The listing builds one solid part. Answer for the finished solid, in the listing's coordinates (mm). Face numbers are marked on the shaded views. A direction names the side the tool comes from. Coordinates: 2 decimals unless noted, no trailing zeros. Write each loop counter-clockwise with the first axis right and the second up, starting at its lowest first coordinate (ties: lowest second). Pieces come first, ordered by that corner, then holes. Notation, with made-up numbers: M 50,56 L 59,56 A29 ccw 59,76 Z; hole C 73,46 d4. An arc over 180 degrees is marked long. Answer as a JSON object with one key per item and string values. Group by question number.
from build123d import *

# Parameters (mm, degrees)
F1_DEPTH  = 2
F2_DEPTH  = 45.5
F4_DEPTH  = 5
F5_R      = 2
F6_R      = 5
F8_DEPTH  = 42.5
F9_R      = 3
F10_DEPTH = 47.501


with BuildPart() as f1:
    # F0 (on Top) → F1 (new body)
    with BuildSketch(Plane.XY):
        with BuildLine():
            ThreePointArc((4.2311346427, 10), (0, 13.850000456), (-4.2311346427, 10))
            Line((-4.2311346427, 10), (-3.2252907411, 10))
            ThreePointArc((-3.2252907411, 10), (0, 12.850000456), (3.2252907411, 10))
            Line((3.2252907411, 10), (4.2311346427, 10))
        make_face()
        with BuildLine():
            Line((3.2252907411, 10), (-3.2252907411, 10))
            ThreePointArc((-3.2252907411, 10), (-0.2003810013, 6.3561836525), (3.25, 9.600000456))
            ThreePointArc((3.25, 9.600000456), (3.2438168034, 9.8003814573), (3.2252907411, 10))
        make_face()
        with BuildLine():
            ThreePointArc((3.2252907411, 10), (0, 12.850000456), (-3.2252907411, 10))
            Line((-3.2252907411, 10), (3.2252907411, 10))
        make_face()
        with BuildLine():
            ThreePointArc((-2.9352384841, 6), (-0.7731344117, 3.3397464334), (0, 0))
            ThreePointArc((0, 0), (0.7731344117, 3.3397464334), (2.9352384841, 6))
            Line((2.9352384841, 6), (2.2588706729, 6))
            ThreePointArc((2.2588706729, 6), (0, 5.350000456), (-2.2588706729, 6))
            Line((-2.2588706729, 6), (-2.9352384841, 6))
        make_face()
        with BuildLine():
            ThreePointArc((2.9352384841, -6), (0.7731344117, -3.3397464334), (0, 0))
            ThreePointArc((0, 0), (-0.7731344117, -3.3397464334), (-2.9352384841, -6))
            Line((-2.9352384841, -6), (2.9352384841, -6))
        make_face()
        with BuildLine():
            ThreePointArc((-4.2311346427, 10), (-3.8118292524, 7.7205170826), (-2.2588706729, 6))
            Line((-2.2588706729, 6), (2.2588706729, 6))
            ThreePointArc((2.2588706729, 6), (3.7190523228, 7.543024564), (4.25, 9.600000456))
            ThreePointArc((4.25, 9.600000456), (4.2452810408, 9.8002225432), (4.2311346427, 10))
            Line((4.2311346427, 10), (3.2252907411, 10))
            ThreePointArc((3.2252907411, 10), (3.2438168034, 9.8003814573), (3.25, 9.600000456))
            ThreePointArc((3.25, 9.600000456), (-0.2003810013, 6.3561836525), (-3.2252907411, 10))
            Line((-3.2252907411, 10), (-4.2311346427, 10))
        make_face()
        with BuildLine():
            ThreePointArc((-2.9352384841, -6), (-0.7731344117, -3.3397464334), (0, 0))
            ThreePointArc((0, 0), (-0.7731344117, 3.3397464334), (-2.9352384841, 6))
            ThreePointArc((-2.9352384841, 6), (-14.6584577236, 2.8174766307), (-8.3490864524, -7.5629934211))
            ThreePointArc((-8.3490864524, -7.5629934211), (-7.6, -6.85), (-6.8509135476, -7.5629934211))
            ThreePointArc((-6.8509135476, -7.5629934211), (-4.7825233693, -7.0584577236), (-2.9352384841, -6))
        make_face()
        with BuildLine():
            ThreePointArc((2.9352384841, 6), (0.7731344117, 3.3397464334), (0, 0))
            ThreePointArc((0, 0), (0.7731344117, -3.3397464334), (2.9352384841, -6))
            ThreePointArc((2.9352384841, -6), (4.7825233693, -7.0584577236), (6.8509135476, -7.5629934211))
            ThreePointArc((6.8509135476, -7.5629934211), (7.6, -6.85), (8.3490864524, -7.5629934211))
            ThreePointArc((8.3490864524, -7.5629934211), (13.2326306926, -5.1023006067), (15.2, 0))
            ThreePointArc((15.2, 0), (10.9397464334, 6.8268655883), (2.9352384841, 6))
        make_face()
        with BuildLine():
            ThreePointArc((-8.3490864524, -7.5629934211), (-14.6584577236, 2.8174766307), (-2.9352384841, 6))
            Line((-2.9352384841, 6), (-2.2588706729, 6))
            ThreePointArc((-2.2588706729, 6), (-3.8118292524, 7.7205170826), (-4.2311346427, 10))
            Line((-4.2311346427, 10), (-17.5, 10))
            Line((-17.5, 10), (-17.5, -10))
            Line((-17.5, -10), (17.5, -10))
            Line((17.5, -10), (17.5, 10))
            Line((17.5, 10), (4.2311346427, 10))
            ThreePointArc((4.2311346427, 10), (4.2452810408, 9.8002225432), (4.25, 9.600000456))
            ThreePointArc((4.25, 9.600000456), (3.7190523228, 7.543024564), (2.2588706729, 6))
            Line((2.2588706729, 6), (2.9352384841, 6))
            ThreePointArc((2.9352384841, 6), (10.9397464334, 6.8268655883), (15.2, 0))
            ThreePointArc((15.2, 0), (13.2326306926, -5.1023006067), (8.3490864524, -7.5629934211))
            ThreePointArc((8.3490864524, -7.5629934211), (8.3497715783, -7.5814910734), (8.35, -7.6))
            ThreePointArc((8.35, -7.6), (7.5814910734, -8.3497715783), (6.8509135476, -7.5629934211))
            ThreePointArc((6.8509135476, -7.5629934211), (4.7825233693, -7.0584577236), (2.9352384841, -6))
            Line((2.9352384841, -6), (-2.9352384841, -6))
            ThreePointArc((-2.9352384841, -6), (-4.7825233693, -7.0584577236), (-6.8509135476, -7.5629934211))
            ThreePointArc((-6.8509135476, -7.5629934211), (-6.8502284217, -7.5814910734), (-6.85, -7.6))
            ThreePointArc((-6.85, -7.6), (-7.6185089266, -8.3497715783), (-8.3490864524, -7.5629934211))
        make_face()
        with BuildLine():
            ThreePointArc((-6.8509135476, -7.5629934211), (-7.6, -6.85), (-8.3490864524, -7.5629934211))
            ThreePointArc((-8.3490864524, -7.5629934211), (-7.6, -7.6), (-6.8509135476, -7.5629934211))
        make_face()
        with BuildLine():
            ThreePointArc((-6.8509135476, -7.5629934211), (-7.6, -7.6), (-8.3490864524, -7.5629934211))
            ThreePointArc((-8.3490864524, -7.5629934211), (-7.6185089266, -8.3497715783), (-6.85, -7.6))
            ThreePointArc((-6.85, -7.6), (-6.8502284217, -7.5814910734), (-6.8509135476, -7.5629934211))
        make_face()
        with BuildLine():
            ThreePointArc((8.3490864524, -7.5629934211), (7.6, -6.85), (6.8509135476, -7.5629934211))
            ThreePointArc((6.8509135476, -7.5629934211), (7.6, -7.6), (8.3490864524, -7.5629934211))
        make_face()
        with BuildLine():
            ThreePointArc((8.3490864524, -7.5629934211), (7.6, -7.6), (6.8509135476, -7.5629934211))
            ThreePointArc((6.8509135476, -7.5629934211), (7.5814910734, -8.3497715783), (8.35, -7.6))
            ThreePointArc((8.35, -7.6), (8.3497715783, -7.5814910734), (8.3490864524, -7.5629934211))
        make_face()
        with BuildLine():
            Line((2.2588706729, 6), (-2.2588706729, 6))
            ThreePointArc((-2.2588706729, 6), (0, 5.350000456), (2.2588706729, 6))
        make_face()
    extrude(amount=-F1_DEPTH)

    # F0 (on Top) → F2 (join)
    with BuildSketch(Plane.XY):
        with BuildLine():
            ThreePointArc((-8.3490864524, -7.5629934211), (-14.6584577236, 2.8174766307), (-2.9352384841, 6))
            Line((-2.9352384841, 6), (-2.2588706729, 6))
            ThreePointArc((-2.2588706729, 6), (-3.8118292524, 7.7205170826), (-4.2311346427, 10))
            Line((-4.2311346427, 10), (-17.5, 10))
            Line((-17.5, 10), (-17.5, -10))
            Line((-17.5, -10), (17.5, -10))
            Line((17.5, -10), (17.5, 10))
            Line((17.5, 10), (4.2311346427, 10))
            ThreePointArc((4.2311346427, 10), (4.2452810408, 9.8002225432), (4.25, 9.600000456))
            ThreePointArc((4.25, 9.600000456), (3.7190523228, 7.543024564), (2.2588706729, 6))
            Line((2.2588706729, 6), (2.9352384841, 6))
            ThreePointArc((2.9352384841, 6), (10.9397464334, 6.8268655883), (15.2, 0))
            ThreePointArc((15.2, 0), (13.2326306926, -5.1023006067), (8.3490864524, -7.5629934211))
            ThreePointArc((8.3490864524, -7.5629934211), (8.3497715783, -7.5814910734), (8.35, -7.6))
            ThreePointArc((8.35, -7.6), (7.5814910734, -8.3497715783), (6.8509135476, -7.5629934211))
            ThreePointArc((6.8509135476, -7.5629934211), (4.7825233693, -7.0584577236), (2.9352384841, -6))
            Line((2.9352384841, -6), (-2.9352384841, -6))
            ThreePointArc((-2.9352384841, -6), (-4.7825233693, -7.0584577236), (-6.8509135476, -7.5629934211))
            ThreePointArc((-6.8509135476, -7.5629934211), (-6.8502284217, -7.5814910734), (-6.85, -7.6))
            ThreePointArc((-6.85, -7.6), (-7.6185089266, -8.3497715783), (-8.3490864524, -7.5629934211))
        make_face()
        with BuildLine():
            ThreePointArc((4.2311346427, 10), (0, 13.850000456), (-4.2311346427, 10))
            Line((-4.2311346427, 10), (-3.2252907411, 10))
            ThreePointArc((-3.2252907411, 10), (0, 12.850000456), (3.2252907411, 10))
            Line((3.2252907411, 10), (4.2311346427, 10))
        make_face()
        with BuildLine():
            ThreePointArc((-4.2311346427, 10), (-3.8118292524, 7.7205170826), (-2.2588706729, 6))
            Line((-2.2588706729, 6), (2.2588706729, 6))
            ThreePointArc((2.2588706729, 6), (3.7190523228, 7.543024564), (4.25, 9.600000456))
            ThreePointArc((4.25, 9.600000456), (4.2452810408, 9.8002225432), (4.2311346427, 10))
            Line((4.2311346427, 10), (3.2252907411, 10))
            ThreePointArc((3.2252907411, 10), (3.2438168034, 9.8003814573), (3.25, 9.600000456))
            ThreePointArc((3.25, 9.600000456), (-0.2003810013, 6.3561836525), (-3.2252907411, 10))
            Line((-3.2252907411, 10), (-4.2311346427, 10))
        make_face()
    extrude(amount=F2_DEPTH)

    # F3 (on face) → F4 (cut)
    with BuildSketch(Plane.XY.offset(45.5)):
        with BuildLine():
            ThreePointArc((4.2311346427, 10), (0, 13.850000456), (-4.2311346427, 10))
            Line((-4.2311346427, 10), (-17.5, 10))
            Line((-17.5, 10), (-17.5, -10))
            Line((-17.5, -10), (17.5, -10))
            Line((17.5, -10), (17.5, 10))
            Line((17.5, 10), (4.2311346427, 10))
        make_face()
        with BuildLine():
            Line((3.6523963674, 8.75), (16.25, 8.75))
            Line((16.25, 8.75), (16.25, -8.75))
            Line((16.25, -8.75), (-16.25, -8.75))
            Line((-16.25, -8.75), (-16.25, 8.75))
            Line((-16.25, 8.75), (-3.6523963674, 8.75))
            ThreePointArc((-3.6523963674, 8.75), (-0.4277929535, 13.3255196398), (3.75, 9.600000456))
            ThreePointArc((3.75, 9.600000456), (3.7255191838, 9.1722075025), (3.6523963674, 8.75))
        make_face(mode=Mode.SUBTRACT)
    extrude(amount=-F4_DEPTH, mode=Mode.SUBTRACT)

    # F5
    f5_edges = [f1.edges().sort_by_distance(p)[0] for p in [
        (17.5, -10, 19.25),
        (17.5, 10, 19.25),
        (-17.5, 10, 19.25),
        (-17.5, -10, 19.25),
    ]]
    fillet(f5_edges, radius=F5_R)

    # F6
    f6_edges = [f1.edges().sort_by_distance(p)[0] for p in [
        (16.25, -8.75, 43),
        (16.25, 8.75, 43),
        (-16.25, 8.75, 43),
        (-16.25, -8.75, 43),
    ]]
    fillet(f6_edges, radius=F6_R)

    # F7 (on face) → F8 (join)
    with BuildSketch(Plane(origin=(0, 0, -2), x_dir=(1, 0, 0), z_dir=(0, 0, -1))):
        with BuildLine():
            ThreePointArc((17.5, 0), (21.5, 4), (25.5, 0))
            ThreePointArc((25.5, 0), (25.0480433512, -1.8469944174), (23.794305811, -3.2766081312))
            ThreePointArc((23.794305811, -3.2766081312), (25.0884620929, -3.1917847095), (25.7612762908, -4.3005482325))
            ThreePointArc((25.7612762908, -4.3005482325), (25.6200398184, -4.8777340259), (25.2282467868, -5.3244883225))
            ThreePointArc((25.2282467868, -5.3244883225), (27.2655704017, -3.0013660128), (28, 0))
            ThreePointArc((28, 0), (24.3504385627, 5.8416607228), (17.5, 5.123475383))
            Line((17.5, 5.123475383), (17.5, 0))
        make_face()
        with BuildLine():
            ThreePointArc((25.7612762908, -4.3005482325), (25.0884620929, -3.1917847095), (23.794305811, -3.2766081312))
            ThreePointArc((23.794305811, -3.2766081312), (23.4873361952, -5.0175187204), (25.2282467868, -5.3244883225))
            ThreePointArc((25.2282467868, -5.3244883225), (25.6200398184, -4.8777340259), (25.7612762908, -4.3005482325))
        make_face()
    extrude(amount=-F8_DEPTH)

    # F9 (on face) → F10 (cut, through all)
    with BuildSketch(Plane(origin=(0, 0, -2), x_dir=(1, 0, 0), z_dir=(0, 0, -1))):
        with Locations((0, -9.600000456)):
            Circle(F9_R)
    extrude(amount=-F10_DEPTH, mode=Mode.SUBTRACT)


solid = f1.part
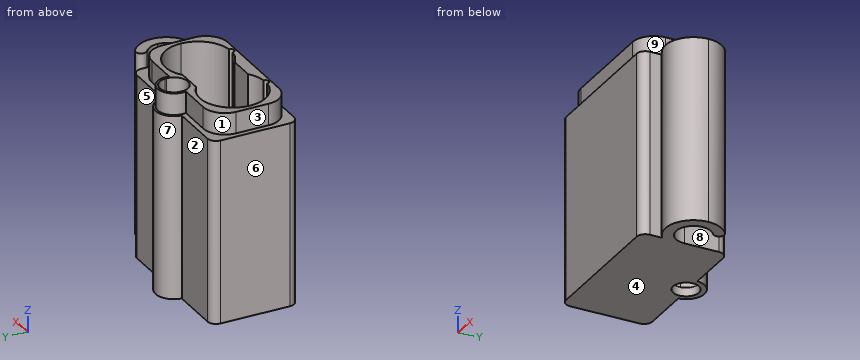
Item 1: A tool of negligible diameter and unlimited length cuts with its end or side. For the marked faces 1, 2, 3, 4 and 5, from which of +Z, -Z, +X, -X, +Y, -Y can it reach the whole face along a straight path? Write none if from no direction.
Item 2: A cutting plane is placed at D-D, the plane x = 21.5. Write down the section's boundary in (y, z).
Item 3: A cutting plane is placed at A-A, the plane x = 7.6. Write down the section's boundary in (y, z).
Item 4: A cutting plane is placed at B-B, the plane z = 30.5. Write down the section's boundary in (x, y), and give its area (3 significant figures).
Item 5: A cutting plane is placed at C-C, the plane x = 13. Write down the section's boundary in (y, z), and give its area (3 significant figures).
Item 6: For a pull along X with two mould halves and no side action, classify the marked faces 6, 7, 8 and 9 as +X half, -X half, draft (parallel to the pull), parting line (faces both ways), or undercut.
Item 7: Consider L1, parallel to Y at x = 0, z = 29; L2, parallel to Y at x = -7.6, z = 14.5; L3, parallel to X at y = 1.5, z = 30. Determine where each line is inside the solid, lowest interval first. Write a range as from..to.
Item 8: Flat-ended cylindrical pins translate along their axes: pin 1 Ø12.5 at (x, z) = (-12, 23) entering from +Y; pin 2 Ø5 at (x, y) = (0, 10) entering from +Z; pin 3 Ø2.5 at (y, z) = (0.5, 43.5) entering from -X; pin 4 Ø8 at (y, z) = (5, 20.5) entering from +X. Find the tip coordinate at first contact, or state that the pin passes through.
Answer:
{
 "1": {"face 1": "+Z, -X, +Y", "face 2": "+Z, -Z, -X, +Y", "face 3": "+Z, -X, +Y, -Y", "face 4": "-Z, +X, -X, +Y, -Y", "face 5": "+Z, -Z, +X, +Y"},
 "2": {"outline": "M -6.5,-2 L -4,-2 L -4,40.5 L -6.5,40.5 Z"},
 "3": {"outline": "M -10,-2 L 10,-2 L 10,40.5 L 8.75,40.5 L 8.75,45.5 L 7.6,45.5 L 7.6,0 L -8.35,0 L -8.35,45.5 L -8.75,45.5 L -8.75,40.5 L -10,40.5 Z"},
 "4": {"outline": "M -17.5,-8 A2 ccw -15.5,-10 L 15.5,-10 A2 ccw 17.5,-8 L 17.5,-5.12 A6.5 ccw long 25.23,5.32 A1.25 ccw 23.79,3.28 A4 cw long 17.5,0 L 17.5,8 A2 ccw 15.5,10 L 4.23,10 A4.25 ccw -4.23,10 L -15.5,10 A2 ccw -17.5,8 Z; hole M -8.35,-7.56 A0.75 ccw long -6.85,-7.56 A7.6 ccw -2.94,-6 L 2.94,-6 A7.6 ccw 6.85,-7.56 A0.75 ccw long 8.35,-7.56 A7.6 ccw long 2.94,6 L -2.94,6 A7.6 ccw long Z; hole C 0,9.6 d6.5", "area": "350 mm2"},
 "5": {"outline": "M -10,-2 L 10,-2 L 10,40.5 L 8.43,40.5 L 8.43,45.5 L 5.35,45.5 L 5.35,0 L -5.35,0 L -5.35,45.5 L -8.43,45.5 L -8.43,40.5 L -10,40.5 Z", "area": "448 mm2"},
 "6": {"face 6": "-X half", "face 7": "parting line", "face 8": "undercut", "face 9": "+X half"},
 "7": {"L1": "-10..-6, 6..6.35, 12.85..13.85", "L2": "-10..-8.35, 7.6..10", "L3": "-17.5..-15.05, 15.05..17.5, 25.21..27.82"},
 "8": {"pin 1": "y = 10", "pin 2": "through", "pin 3": "x = -16.25", "pin 4": "x = 27.92"}
}
